Autodesk Inventor part; units mm, degrees
ref_plane "YZ Plane" through (0, 0, 0) normal (1, 0, 0) x (0, 1, 0)
ref_plane "XZ Plane" through (0, 0, 0) normal (0, 1, 0) x (-1, 0, 0)
ref_plane "XY Plane" through (0, 0, 0) normal (0, 0, 1) x (1, 0, 0)
sketch "Sketch1" plane through (0, 0, 0) normal (0, 0, 1) x (1, 0, 0)
  circle A0 centre (0, 0) radius 25.4
  dimension "d0" = 50.8
extrude "Extrusion1" add sketch "Sketch1" along normal mid plane 9.525
sketch "Sketch3" plane through (0, 0, 4.7625) normal (0, 0, 1) x (1, 0, 0)
  circle A0 centre (0, 0) radius 25.4
  line L0 (-2.8374, 21.892) -> (-2.8374, 21.8722)
  arc A1 (3.8096, 25.1127) -> (-2.8374, 25.241) centre (0, 0) ccw
  arc A2 (3.3133, 21.8251) -> (-2.466, 21.937) centre (0, 0) ccw
  line L1 (3.3133, 21.8251) -> (3.8096, 25.1127)
  line L2 (-2.466, 21.937) -> (-2.8374, 25.241)
  dimension "d17" = 3.3249
  dimension "d24" = 15
extrude "Extrusion4" cut sketch "Sketch3" against normal blind 9.525 contours L1 A2 L2 A0 picked at (-1.9747, 24.1901)
pattern_circular "Circular Pattern2" count 12 over 360 about axis through (0, 0, -10) along (0, 0, 1) of "Extrusion4"
sketch "Sketch4" plane through (0, 0, -4.7625) normal (0, 0, -1) x (-1, 0, 0)
  circle A0 centre (0, 0) radius 12.7
  dimension "d27" = 25.4
extrude "Extrusion5" add sketch "Sketch4" along normal blind 12.7
sketch "Sketch2" plane through (0, 0, 4.7625) normal (0, 0, 1) x (1, 0, 0)
  line L0 (7.3323, 0) -> (3.6662, -6.35)
  line L1 (3.6662, -6.35) -> (-3.6662, -6.35)
  line L2 (-3.6662, -6.35) -> (-7.3323, 0)
  line L3 (-7.3323, 0) -> (-3.6662, 6.35)
  line L4 (-3.6662, 6.35) -> (3.6662, 6.35)
  line L5 (3.6662, 6.35) -> (7.3323, 0)
  point P0 (0, 0)
  point P1 (0, 0)
  dimension "d23" = 12.7
extrude "Extrusion2" cut sketch "Sketch2" against normal through all
equation "\"d0\" = externalDiameter"
equation "\"d1\" = thickness"
equation "\"d17\" = heightOfSpline"
equation "\"d18\" = thickness"
equation "\"d23\" = shaftHexSize"
equation "\"externalDiameter\" = 50.8"
equation "\"thickness\" = 9.525"
equation "\"shaftHexSize\" = 12.7"
equation "\"pi\" = 3.141593"
properties part number "centerPartOfLock" material "PC/ABS Plastic"
Design review of the part built by this model. Coordinates are the model's own, in mm. A direction names the side the tool comes from. Coordinates: 2 decimals unless noted, no trailing zeros. Write each loop counter-clockwise with the first axis right and the second up, starting at its lowest first coordinate (ties: lowest second). Pieces come first, ordered by that corner, then holes. Notation, with made-up numbers: (76, 56) - (130, 56) arc R21 ccw to (130, 94) - close; hole circle Ø6 at (-40, -29.75). An arc over 180 degrees is marked (long way). Use one line per item in the form item = value.
Q1. Consider section B-B (z = -5.5). Write out the cut boundary in (x, y), plus the area to 3 significant figures.
Taken from the geometry:
outline = circle Ø25.4 at (0, 0); hole (-7.33, 0) - (-3.67, -6.35) - (3.67, -6.35) - (7.33, 0) - (3.67, 6.35) - (-3.67, 6.35) - close
area = 367 mm^2
Q2. The part is to be moulded in two halves that separate along Y. For faces 1 (the flat face through (-3.56, -23.45, 0.07)), 2 (the flat face through (-18.526, 14.804, 0.067)), 3 (the cylindrical face through (2.75, 12.4, -11.02)), say which applies: +Y half, -Y half, draft (parallel to the pull), parting line (faces both ways), or undercut.
Taken from the geometry:
face_1 = -Y half
face_2 = undercut
face_3 = parting line
Q3. For probe 1 along X at (y, z) = (-18.5, 0.5); probe 2 along Z at (x, y) = (-10, 12.5); probe 3 along X at (y, z) = (-6, -5.75), list the stretches that pass through material, from the lowest coordinate up.
Taken from the geometry:
probe_1 = -17.4 to -14.78, -12.04 to 12.04, 13.65 to 17.4
probe_2 = -4.76 to 4.76
probe_3 = -11.19 to -3.87, 3.87 to 11.19
Q4. Insertion check: pin 1 Ø5 at (x, z) = (-1.5, -12) entering from -Y; pin 2 Ø1 at (x, z) = (11, -8.5) entering from -Y; pin 3 Ø5 at (x, y) = (-20, 20) entering from -Z (1 decimal); pin 4 Ø4 at (y, z) = (14.5, -4) entering from -X. Each pin has a flat end and moves straight along its axis. Give the tip position at first contact, or say it passes through.
Taken from the geometry:
pin_1 = -12.7
pin_2 = -7.14
pin_3 = through
pin_4 = -19.84
Q5. Consider section C-C (y = -5.5). Write out the cut boundary in (x, z), plus the area to 3 significant figures.
Taken from the geometry:
outline = (-24.8, -4.76) - (-11.45, -4.76) - (-11.45, -17.46) - (-4.16, -17.46) - (-4.16, 4.76) - (-24.8, 4.76) - close; (4.16, -17.46) - (11.45, -17.46) - (11.45, -4.76) - (24.8, -4.76) - (24.8, 4.76) - (4.16, 4.76) - close
area = 578 mm^2
Q6. Machinability: for faces 4 (the flat face through (5.474, 3.219, -6.194)), 5 (the flat face through (-19.084, -14.077, 0.067)), 6 (the flat face through (14.077, -19.084, 0.067)), which of the approach directions +Z, -Z, +X, -X, +Y, -Y give a long, thin tool a straight path to every point of the face, cutting with its end or side? Answer none if there is none.
Taken from the geometry:
face_4 = +Z, -Z
face_5 = +Z, -Z, -X
face_6 = +Z, -Z, -Y
Q7. Consider section D-D (x = -12). Write out the cut boundary in (y, z).
Taken from the geometry:
outline = (-18.53, -4.76) - (-4.16, -4.76) - (-4.16, -17.46) - (4.16, -17.46) - (4.16, -4.76) - (18.53, -4.76) - (18.53, 4.76) - (-18.53, 4.76) - close
Q8. Consider section A-A (x = 0). Write out the cut boundary in (y, z), plus the area to 3 significant figures.
Taken from the geometry:
outline = (-22.08, -4.76) - (-12.7, -4.76) - (-12.7, -17.46) - (-6.35, -17.46) - (-6.35, 4.76) - (-22.08, 4.76) - close; (6.35, -17.46) - (12.7, -17.46) - (12.7, -4.76) - (22.08, -4.76) - (22.08, 4.76) - (6.35, 4.76) - close
area = 461 mm^2
